```python
from build123d import *

# Parameters (mm, degrees)
SKETCH1_R           = 1.1
SKETCH1_R_2         = 1.5
BOSS_EXTRUDE1_DEPTH = 3.048
SKETCH2_R           = 3.1
SKETCH2_R_2         = 1.1
BOSS_EXTRUDE2_DEPTH = 5
BOSS_EXTRUDE4_START = -13.75
SKETCH1_5_R         = 1.1
SKETCH1_5_R_2       = 1.5
BOSS_EXTRUDE4_DEPTH = 13.75
CUT_EXTRUDE1_DEPTH  = 113.753315675
CUT_EXTRUDE2_REACH  = 72.409
FILLET1_R           = 5
BOSS_EXTRUDE6_DEPTH = 1.5


with BuildPart() as part:
    # Sketch1 → Boss-Extrude1 (new body)
    with BuildSketch(Plane(origin=(0, 0, 0), x_dir=(1, 0, 0), z_dir=(0, 1, 0))):
        with BuildLine():
            Line((-40.209744398, 44.711958299), (28.240255602, 44.711958299))
            ThreePointArc((28.240255602, 44.711958299), (44.41885963, 38.010560578), (51.120255602, 21.831955824))
            Line((51.120255602, 21.831955824), (51.120255602, -34.598189146))
            ThreePointArc((51.120255602, -34.598189146), (47.776738906, -42.160841434), (40.130306185, -45.308043388))
            Line((40.130306185, -45.308043388), (-40.209744398, -45.308043388))
            ThreePointArc((-40.209744398, -45.308043388), (-47.987919588, -42.086217385), (-51.209744398, -34.308041701))
            Line((-51.209744398, -34.308041701), (-51.209744398, 33.711958299))
            ThreePointArc((-51.209744398, 33.711958299), (-47.987918991, 41.490132892), (-40.209744398, 44.711958299))
        make_face()
        with Locations(Location((-39.019744398, -34.478043388, 0), (0, 0, 90))):
            Circle(SKETCH1_R, mode=Mode.SUBTRACT)
        with Locations(Location((-18.179744398, -34.478043388, 0), (0, 0, 90))):
            Circle(SKETCH1_R, mode=Mode.SUBTRACT)
        with Locations(Location((-39.019744398, 33.731958299, 0), (0, 0, 90))):
            Circle(SKETCH1_R, mode=Mode.SUBTRACT)
        with Locations(Location((8.610255602, 33.731915189, 0), (0, 0, 90))):
            Circle(SKETCH1_R, mode=Mode.SUBTRACT)
        with Locations(Location((8.655, 10.511958299, 0), (0, 0, 90))):
            Circle(SKETCH1_R, mode=Mode.SUBTRACT)
        with Locations(Location((-45.866598648, 39.368812549, 0), (0, 0, 90))):
            Circle(SKETCH1_R_2, mode=Mode.SUBTRACT)
        with Locations(Location((42.297539172, 35.889240349, 0), (0, 0, 90))):
            Circle(SKETCH1_R_2, mode=Mode.SUBTRACT)
        with Locations(Location((45.695011225, -40.000653974, 0), (0, 0, 90))):
            Circle(SKETCH1_R_2, mode=Mode.SUBTRACT)
        with Locations(Location((-45.858259021, -39.973270185, 0), (0, 0, 90))):
            Circle(SKETCH1_R_2, mode=Mode.SUBTRACT)
    extrude(amount=BOSS_EXTRUDE1_DEPTH)

    # Sketch2 → Boss-Extrude2 (add)
    # profile 1 of 7: a face of its own
    with BuildSketch(Plane(origin=(0, 3.048, 0), x_dir=(1, 0, 0), z_dir=(0, 1, 0))):
        with Locations(Location((-39.019744398, 33.731958299, 0), (0, 0, 270))):
            Circle(SKETCH2_R)
        with Locations(Location((-39.019744398, 33.731958299, 0), (0, 0, 90))):
            Circle(SKETCH2_R_2, mode=Mode.SUBTRACT)
    # profile 2 of 7: a face of its own
    with BuildSketch(Plane(origin=(0, 3.048, 0), x_dir=(1, 0, 0), z_dir=(0, 1, 0))):
        with Locations(Location((8.610255602, 33.731915189, 0), (0, 0, 270))):
            Circle(SKETCH2_R)
        with Locations(Location((8.610255602, 33.731915189, 0), (0, 0, 90))):
            Circle(SKETCH2_R_2, mode=Mode.SUBTRACT)
    # profile 3 of 7: a face of its own
    with BuildSketch(Plane(origin=(0, 3.048, 0), x_dir=(1, 0, 0), z_dir=(0, 1, 0))):
        with Locations(Location((8.655, 10.511958299, 0), (0, 0, 270))):
            Circle(SKETCH2_R)
        with Locations(Location((8.655, 10.511958299, 0), (0, 0, 90))):
            Circle(SKETCH2_R_2, mode=Mode.SUBTRACT)
    # profile 4 of 7: a face of its own
    with BuildSketch(Plane(origin=(0, 3.048, 0), x_dir=(1, 0, 0), z_dir=(0, 1, 0))):
        with Locations(Location((-18.179744398, -34.478043388, 0), (0, 0, 270))):
            Circle(SKETCH2_R)
        with Locations(Location((-18.179744398, -34.478043388, 0), (0, 0, 90))):
            Circle(SKETCH2_R_2, mode=Mode.SUBTRACT)
    # profile 5 of 7: a face of its own
    with BuildSketch(Plane(origin=(0, 3.048, 0), x_dir=(1, 0, 0), z_dir=(0, 1, 0))):
        with Locations(Location((-39.019744398, -34.478043388, 0), (0, 0, 270))):
            Circle(SKETCH2_R)
        with Locations(Location((-39.019744398, -34.478043388, 0), (0, 0, 90))):
            Circle(SKETCH2_R_2, mode=Mode.SUBTRACT)
    # profile 6 of 7: a face of its own
    with BuildSketch(Plane(origin=(0, 3.048, 0), x_dir=(1, 0, 0), z_dir=(0, 1, 0))):
        with Locations(Location((39.720255602, -34.478043388, 0), (0, 0, 270))):
            Circle(SKETCH2_R)
    # profile 7 of 7: a face of its own
    with BuildSketch(Plane(origin=(0, 3.048, 0), x_dir=(1, 0, 0), z_dir=(0, 1, 0))):
        with Locations(Location((39.720255602, 10.511958299, 0), (0, 0, 270))):
            Circle(SKETCH2_R)
    extrude(amount=BOSS_EXTRUDE2_DEPTH)

    # Sketch1_5 → Boss-Extrude4 (add)
    with BuildSketch(Plane(origin=(0, 0, 0), x_dir=(1, 0, 0), z_dir=(0, 1, 0)).offset(BOSS_EXTRUDE4_START)):
        with BuildLine():
            Line((-40.209744398, 44.711958299), (28.240255602, 44.711958299))
            ThreePointArc((28.240255602, 44.711958299), (44.41885963, 38.010560578), (51.120255602, 21.831955824))
            Line((51.120255602, 21.831955824), (51.120255602, -34.598189146))
            ThreePointArc((51.120255602, -34.598189146), (47.776738906, -42.160841434), (40.130306185, -45.308043388))
            Line((40.130306185, -45.308043388), (-40.209744398, -45.308043388))
            ThreePointArc((-40.209744398, -45.308043388), (-47.987919588, -42.086217385), (-51.209744398, -34.308041701))
            Line((-51.209744398, -34.308041701), (-51.209744398, 33.711958299))
            ThreePointArc((-51.209744398, 33.711958299), (-47.987918991, 41.490132892), (-40.209744398, 44.711958299))
        make_face()
        with Locations(Location((-39.019744398, -34.478043388, 0), (0, 0, 90))):
            Circle(SKETCH1_5_R, mode=Mode.SUBTRACT)
        with Locations(Location((-18.179744398, -34.478043388, 0), (0, 0, 90))):
            Circle(SKETCH1_5_R, mode=Mode.SUBTRACT)
        with Locations(Location((-39.019744398, 33.731958299, 0), (0, 0, 90))):
            Circle(SKETCH1_5_R, mode=Mode.SUBTRACT)
        with Locations(Location((8.610255602, 33.731915189, 0), (0, 0, 90))):
            Circle(SKETCH1_5_R, mode=Mode.SUBTRACT)
        with Locations(Location((8.655, 10.511958299, 0), (0, 0, 90))):
            Circle(SKETCH1_5_R, mode=Mode.SUBTRACT)
        with Locations(Location((-45.866598648, 39.368812549, 0), (0, 0, 90))):
            Circle(SKETCH1_5_R_2, mode=Mode.SUBTRACT)
        with Locations(Location((42.297539172, 35.889240349, 0), (0, 0, 90))):
            Circle(SKETCH1_5_R_2, mode=Mode.SUBTRACT)
        with Locations(Location((45.695011225, -40.000653974, 0), (0, 0, 90))):
            Circle(SKETCH1_5_R_2, mode=Mode.SUBTRACT)
        with Locations(Location((-45.858259021, -39.973270185, 0), (0, 0, 90))):
            Circle(SKETCH1_5_R_2, mode=Mode.SUBTRACT)
    extrude(amount=BOSS_EXTRUDE4_DEPTH)

    # Sketch3 → Cut-Extrude1 (cut, through all)
    with BuildSketch(Plane.ZY.offset(51.209744398)):
        Polygon((-44.711958299, -13.75), (-33.711958299, -13.75), (34.308041701, -13.75), (45.308043388, -13.75), (45.308043388, -1.898641945), align=None)
    extrude(amount=-CUT_EXTRUDE1_DEPTH, mode=Mode.SUBTRACT)

    # Cut-Extrude2: up to this plane
    cut_extrude2_end = Plane(origin=(51.120255602, -8.792775693, -45.36458926), z_dir=(0, 0.9914448613738103, -0.13052619222005254))
    # Sketch4 → Cut-Extrude2 (cut, up to the surface)
    with BuildSketch(Plane(origin=(0, 3.048, 0), x_dir=(1, 0, 0), z_dir=(0, 1, 0)), mode=Mode.PRIVATE) as cut_extrude2_sk1:
        Polygon((0.790255602, 2.691956612), (41.120255602, 2.691956612), (41.120255602, -27.308043388), (-41.209744398, -27.308043388), (-41.209744398, 2.691956612), (-41.209744398, 25.691956612), (0.790255602, 25.691956612), align=None)
    cut_extrude2_tool1 = split(extrude(cut_extrude2_sk1.sketch, amount=-CUT_EXTRUDE2_REACH, mode=Mode.PRIVATE), bisect_by=cut_extrude2_end, keep=Keep.BOTH, mode=Mode.PRIVATE)
    add(cut_extrude2_tool1.solids().sort_by_distance((-5.714115, 3.048, 4.857594))[0], mode=Mode.SUBTRACT)

    # Fillet1
    fillet1_edges = [part.edges().sort_by_distance(p)[0] for p in [
        (-41.209744398, -1.577412235, -25.691956612),
        (0.790255602, -1.577412235, -25.691956612),
        (0.790255602, -0.063408513, -2.691956612),
        (41.120255602, -0.063408513, -2.691956612),
        (41.120255602, 1.911378951, 27.308043388),
        (-41.209744398, 1.911378951, 27.308043388),
    ]]
    fillet(fillet1_edges, radius=FILLET1_R)

    # Sketch5 → Boss-Extrude6 (add, along a direction that is not the sketch's normal)
    with BuildSketch(Plane(origin=(0, -7.72958688, 1.017619418), x_dir=(1, 0, 0), z_dir=(0, -0.9914448613738103, 0.13052619222005257))):
        with BuildLine():
            Line((-51.209744398, 33.577685726), (-51.209744398, -35.029257874))
            add(Edge.make_bspline(
                [(-51.209744398, -35.029257874), (-51.209744398, -46.124176441), (-40.209744398, -46.124176441)],
                knots=[4.71238898, 4.71238898, 4.71238898, 6.283185307, 6.283185307, 6.283185307], degree=2, weights=[1, 0.707106781, 1]))
            Line((-40.209744398, -46.124176441), (28.240255602, -46.124176441))
            add(Edge.make_bspline(
                [(28.240255602, -46.124176441), (51.120255602, -46.124176441), (51.120255602, -23.046745823)],
                knots=[0, 0, 0, 1.570796327, 1.570796327, 1.570796327], degree=2, weights=[1, 0.707106781, 1]))
            Line((51.120255602, -23.046745823), (51.120255602, 33.87033514))
            add(Edge.make_bspline(
                [(51.120255602, 33.87033514), (50.756477038, 44.58229707), (40.130306185, 44.672604293)],
                knots=[1.605036011, 1.605036011, 1.605036011, 3.133166993, 3.133166993, 3.133166993], degree=2, weights=[1, 0.722029225, 1]))
            Line((40.130306185, 44.672604293), (-40.209744398, 44.672604293))
            add(Edge.make_bspline(
                [(-40.209744398, 44.672604293), (-51.209744398, 44.672604293), (-51.209744398, 33.577685726)],
                knots=[3.141592654, 3.141592654, 3.141592654, 4.71238898, 4.71238898, 4.71238898], degree=2, weights=[1, 0.707106781, 1]))
        make_face()
    extrude(amount=BOSS_EXTRUDE6_DEPTH, dir=(0, -1, 0))


solid = part.part
```
Geometry: final body of the model. Coordinates: model frame, mm. A direction names the side the tool comes from. Give positions to 0.01 mm unless a question says otherwise; leave off trailing zeros. Write each loop counter-clockwise with the first axis right and the second up, starting at its lowest first coordinate (ties: lowest second). Pieces come first, ordered by that corner, then holes.
1. Reachability of faces 1 (the flat face through (-39, 8.048, -32)), 2 (the cylindrical face through (-39.71, 1.89, 25.88)) from +Z, -Z, +X, -X, +Y, -Y: full face, straight path, thin tool, end or side. Return the list, or none.
2. Pin query (flat end, axial travel): P1, Ø5, axis at x = 42.3, z = -35.89, coming from the -Y side; P2, Ø2, axis at x = -39.02, z = 34.48, coming from the +Y side; P3, Ø3, axis at x = 37, z = -25, coming from the +Y side. Return the tip coordinate at first contact, or that it passes through.
3. Section query B-B, the plane x = -29. Return loops of the section in (y, z).
4. Section query A-A, the plane y = 4.25. Count the separate pieces of the cut face and the enclosed holes in it, then the cut area to 3 significant figures.
5. Section query C-C, the plane z = -5.5. Return loops of the section in (x, y).
6. Line query: probe 1 along X at (y, z) = (0.25, -8); probe 2 along X at (y, z) = (-1, -22); probe 3 along Z at (x, y) = (4, 3). Output: solid intervals per line, ascending.
Computed:
1. face 1: +Z, -Z, +X, -X, +Y
1. face 2: +Y
2. P1: stops at y = -14.42
2. P2: stops at y = -3.19
2. P3: stops at y = 3.05
3. outline: (-15.25, -44.71) - (3.05, -44.71) - (3.05, -25.69) - (-6.2, -25.69) - (0.77, 27.31) - (3.05, 27.31) - (3.05, 45.31) - (-3.4, 45.31) - close
4. separate pieces: 7
4. enclosed holes: 5
4. area: 192 mm2
5. outline: (-51.21, -10.09) - (51.12, -10.09) - (51.12, 3.05) - (1.3, 3.05) - (1.3, -3.54) - (-41.21, -3.54) - (-41.21, 3.05) - (-51.21, 3.05) - close
6. probe 1: x = -51.21 to -41.21, 0.79 to 51.12
6. probe 2: x = -51.21 to -41.04, 0.62 to 51.12
6. probe 3: z = -44.71 to -3.02, 27.31 to 45.31
